Here's how the part is built. I have some questions about the finished solid (model axes, mm). Face numbers are marked on the shaded views. A direction names the side the tool comes from. Round coordinates to 2 decimals unless told otherwise and drop trailing zeros. Write each loop counter-clockwise with the first axis right and the second up, starting at its lowest first coordinate (ties: lowest second). Pieces come first, ordered by that corner, then holes. Notation, with made-up numbers: (86.5, -29.5) - (106.5, -29.5) arc R14 cw to (106.5, -2.5) - close; hole circle Ø6 at (36.5, -6.5). An arc over 180 degrees is marked (long way). Return JSON: item names as keys, results as strings. Group by question number.
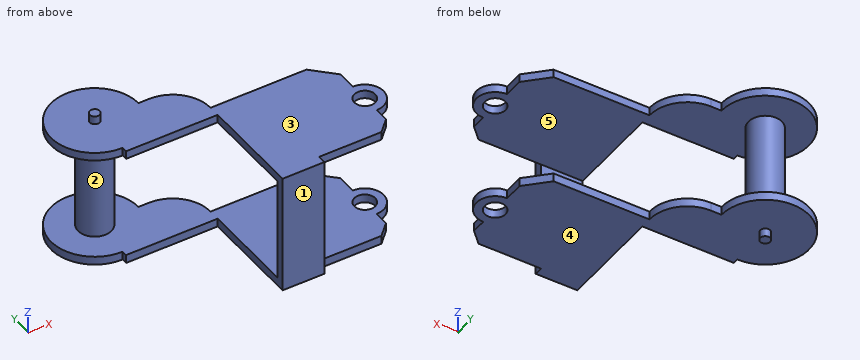
```python
from build123d import *

# Parameters (mm, degrees)
SKETCH_1_R           = 4
SKETCH_1_R_2         = 2.50023196
EXTRUDE_3_DEPTH      = 29
SKETCH_5_W           = 29.813353088
SKETCH_5_H           = 25
CUT_EXTRUDE_2_DEPTH  = 50
SKETCH_6_W           = 25
SKETCH_6_H           = 54.055656888
CUT_EXTRUDE_3_DEPTH  = 50
SKETCH_7_R           = 4
SKETCH_7_R_2         = 1.2
EXTRUDE_4_DEPTH      = 29
SKETCH_10_R          = 1.2
EXTRUDE_5_DEPTH      = 2
EXTRUDE_5_DEPTH_BACK = 31


with BuildPart() as part:
    # 草图1 → 凸台-拉伸3 (new body)
    with BuildSketch(Plane.XY):
        with BuildLine():
            Line((-23.562506416, 27.500198397), (-23.562506416, 27.598880866))
            ThreePointArc((-23.562506416, 27.598880866), (-26.198545385, 33.962841897), (-32.562506416, 36.598880866))
            Line((-32.562506416, 36.598880866), (-35.062506416, 36.598880866))
            ThreePointArc((-35.062506416, 36.598880866), (-52.987127618, 44.023502068), (-45.562506416, 26.098880866))
            Line((-45.562506416, 26.098880866), (-45.562506416, 24.798880866))
            Line((-45.562506416, 24.798880866), (-23.562506416, 24.798880866))
            Line((-23.562506416, 24.798880866), (-23.562506416, 2.297860243))
            Line((-23.562506416, 2.297860243), (-23.562506416, 0.297860243))
            Line((-23.562506416, 0.297860243), (-13.562506416, 0.297860243))
            Line((-13.562506416, 0.297860243), (-13.562506416, 2.297860243))
            Line((-13.562506416, 2.297860243), (1.437493584, 2.297860243))
            Line((1.437493584, 2.297860243), (4.437493584, 5.297860243))
            Line((4.437493584, 5.297860243), (4.437493584, 8.798464088))
            ThreePointArc((4.437493584, 8.798464088), (8.937910362, 13.298880866), (4.437493584, 17.799297644))
            Line((4.437493584, 17.799297644), (4.437493584, 22.500198397))
            Line((4.437493584, 22.500198397), (-0.562506416, 27.500198397))
            Line((-0.562506416, 27.500198397), (-23.562506416, 27.500198397))
        make_face()
        with Locations((-45.562506416, 36.598880866)):
            Circle(SKETCH_1_R, mode=Mode.SUBTRACT)
        with Locations((4.437493584, 13.298880866)):
            Circle(SKETCH_1_R_2, mode=Mode.SUBTRACT)
    extrude(amount=EXTRUDE_3_DEPTH)

    # 草图5 → 切除-拉伸2 (cut)
    with BuildSketch(Plane.XZ.offset(-2.297860243)):
        with Locations((1.344170128, 14.537987409)):
            Rectangle(SKETCH_5_W, SKETCH_5_H)
    extrude(amount=-CUT_EXTRUDE_2_DEPTH, mode=Mode.SUBTRACT)

    # 草图6 → 切除-拉伸3 (cut)
    with BuildSketch(Plane(origin=(-13.562506416, 0, 0), x_dir=(0, 0, -1), z_dir=(1, 0, 0))):
        with Locations((-14.537987409, 29.325688687)):
            Rectangle(SKETCH_6_W, SKETCH_6_H)
    extrude(amount=-CUT_EXTRUDE_3_DEPTH, mode=Mode.SUBTRACT)

    # 草图7 → 凸台-拉伸4 (add)
    with BuildSketch(Plane.XY.offset(29)):
        with Locations((-45.562506416, 36.598880866)):
            Circle(SKETCH_7_R)
        with Locations((-45.562506416, 36.598880866)):
            Circle(SKETCH_7_R_2, mode=Mode.SUBTRACT)
    extrude(amount=-EXTRUDE_4_DEPTH)

    # 草图10 → 凸台-拉伸5 (add, two sides)
    with BuildSketch(Plane(origin=(0, 0, 0), x_dir=(-1, 0, 0), z_dir=(0, 0, -1))) as extrude_5_sk:
        with Locations((45.562506416, 36.598880866)):
            Circle(SKETCH_10_R)
    extrude(amount=EXTRUDE_5_DEPTH)
    extrude(extrude_5_sk.sketch, amount=-EXTRUDE_5_DEPTH_BACK)


solid = part.part
```
1) Imagine slicing it at C-C (z = 22). Please give me the cut outline in (x, y), plus the area to 3 significant figures.
2) Imagine slicing it at D-D (y = 14). Please give me the cut outline in (x, z).
3) I need wall thicknesses on line 1 along Z through (x, y) = (-11, 13); line 2 along Y through (x, z) = (-19, 28); line 3 along Y through (x, z) = (-23, 6). Which ranges of each line are inside material? Lowest first, please.
4) If we mould it in two halves opening along Z, with no side actions, what happens to the marked faces 3, 4 and 5? For each: released by +Z, released by -Z, zero draft, split by the parting line, or undercut.
5) Will these pins go through, and if not, where does the flat tip stop? pin 1 Ø5 at (x, z) = (-2.5, 23) entering from +Y; pin 2 Ø1 at (y, z) = (1, 14) entering from +X; pin 3 Ø0.7 at (y, z) = (25.5, 27.5) entering from -X; pin 4 Ø0.6 at (x, z) = (-40, 27.5) entering from -Y.
6) Imagine slicing it at A-A (y = 21.5). Please give me the cut outline in (x, z).
7) Imagine slicing it at B-B (x = -4). Please give me the cut outline in (y, z).
8) For the marked faces 1 and 2, which set-ups out of +Z, -Z, +X, -X, +Y, -Y let a thin tool reach every point of the face, with its end or its side?
Results found:
{
 "1": {"outline": "circle Ø8 at (-45.56, 36.6); (-23.56, 0.3) - (-13.56, 0.3) - (-13.56, 2.3) - (-23.56, 2.3) - close", "area": "70.3 mm²"},
 "2": {"outline": "(-23.56, 0) - (2.04, 0) - (2.04, 2.04) - (-23.56, 2.04) - close; (-23.56, 27.04) - (2.04, 27.04) - (2.04, 29) - (-23.56, 29) - close; (6.84, 0) - (8.88, 0) - (8.88, 2.04) - (6.84, 2.04) - close; (6.84, 27.04) - (8.88, 27.04) - (8.88, 29) - (6.84, 29) - close"},
 "3": {"line 1": "z = 0 to 2.04, 27.04 to 29", "line 2": "y = 0.3 to 27.5", "line 3": "y = 0.3 to 2.3"},
 "4": {"face 3": "released by +Z", "face 4": "released by -Z", "face 5": "undercut"},
 "5": {"pin 1": "passes through", "pin 2": "stops at x = -13.56", "pin 3": "stops at x = -45.56", "pin 4": "stops at y = 24.8"},
 "6": {"outline": "(-23.56, 0) - (4.44, 0) - (4.44, 2.04) - (-23.56, 2.04) - close; (-23.56, 27.04) - (4.44, 27.04) - (4.44, 29) - (-23.56, 29) - close"},
 "7": {"outline": "(2.3, 0) - (27.5, 0) - (27.5, 2.04) - (2.3, 2.04) - close; (2.3, 27.04) - (27.5, 27.04) - (27.5, 29) - (2.3, 29) - close"},
 "8": {"face 1": "+Z, -Z, +X, -X, -Y", "face 2": "none"}
}
